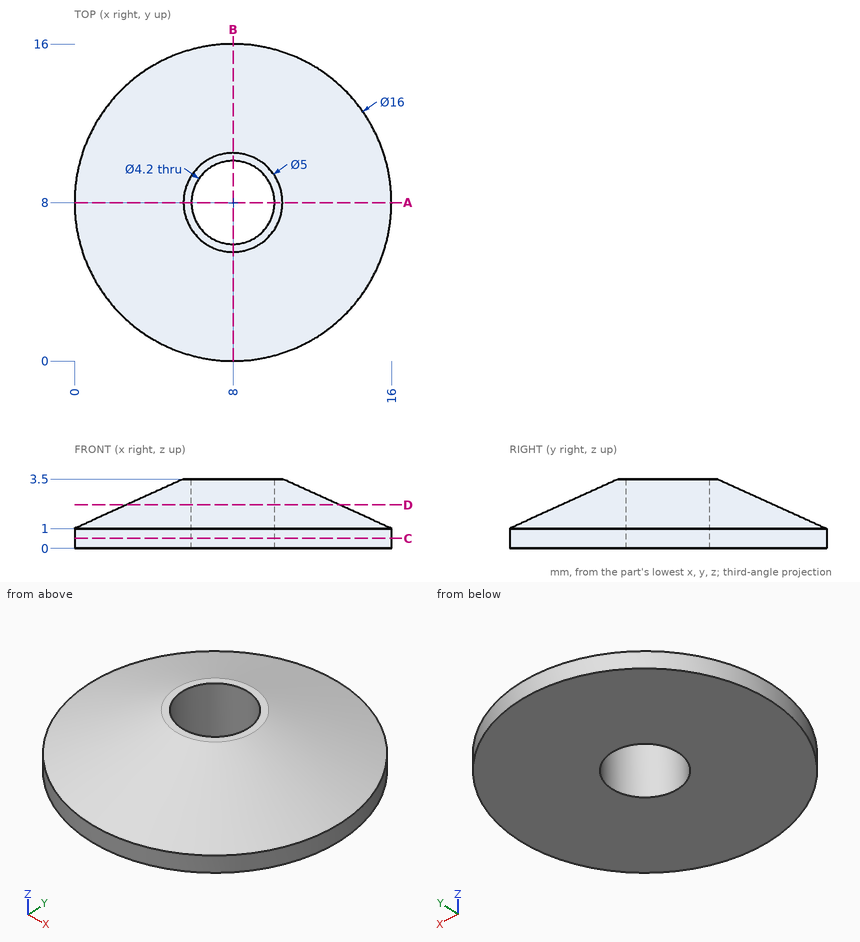
Geometry: see drawing. Coordinates: mm, zero at the bounding-box minimum. Give positions to 0.01 mm unless a question says otherwise; leave off trailing zeros. Write each loop counter-clockwise with the first axis right and the second up, starting at its lowest first coordinate (ties: lowest second). Pieces come first, ordered by that corner, then holes. Notation, with made-up numbers: M -30.5,76 L 8.5,76 A22 cw 8.5,88 Z; hole C 74,-3.5 d8. An arc over 180 degrees is marked long. Answer in a Markdown table with one row per item. Add a question column.
(1) Section A-A on y = 8. Return loops of the section in (x, z).
(2) Section C-C on z = 0.5. Return loops of the section in (x, y).
(3) First-contact query: pin 1 (1.5 mm diameter, centred on y = 13, z = 1, fed in from -X); pin 2 (2 mm diameter, centred on x = 4, z = 0.5, fed in from -Y). Flat tips, straight axial feed; report the tip coordinate or a pass-through.
(4) Ray query, line 1 (Y direction, x = 8, z = 0.8); line 2 (Y direction, x = 8, z = 2.05); line 3 (X direction, y = 8.25, z = 3.15). Return the intervals inside material, ascending.
(5) Section D-D on z = 2.2. Return loops of the section in (x, y), and give its area (3 significant figures).
Result set:
| question | item | result |
|---|---|---|
| 1 | outline | M 0,0 L 5.9,0 L 5.9,3.5 L 5.5,3.5 L 0,1 Z; M 10.1,0 L 16,0 L 16,1 L 10.5,3.5 L 10.1,3.5 Z |
| 2 | outline | C 8,8 d16; hole C 8,8 d4.2 |
| 3 | pin 1 | stops at x = 1.22 |
| 3 | pin 2 | stops at y = 0.58 |
| 4 | line 1 | y = 0 to 5.9, 10.1 to 16 |
| 4 | line 2 | y = 2.31 to 5.9, 10.1 to 13.69 |
| 4 | line 3 | x = 4.74 to 5.91, 10.09 to 11.26 |
| 5 | outline | C 8,8 d10.72; hole C 8,8 d4.2 |
| 5 | area | 76.4 mm^2 |
